from build123d import *

# Parameters (mm, degrees)
SKETCH1_W           = 120
SKETCH1_H           = 48
BOSS_EXTRUDE1_DEPTH = 4
SKETCH2_W           = 14
SKETCH2_H           = 3
BOSS_EXTRUDE2_DEPTH = 5
SKETCH3_R           = 1.7
CUT_EXTRUDE1_DEPTH  = 5
SKETCH4_R           = 3
CUT_EXTRUDE2_DEPTH  = 3


with BuildPart() as part:
    # Sketch1 → Boss-Extrude1 (new body)
    with BuildSketch(Plane(origin=(0, 0, 0), x_dir=(1, 0, 0), z_dir=(0, 1, 0))):
        with Locations((9.738916256, -3.92364532)):
            Rectangle(SKETCH1_W, SKETCH1_H)
    extrude(amount=BOSS_EXTRUDE1_DEPTH)

    # Sketch2 → Boss-Extrude2 (add)
    with BuildSketch(Plane(origin=(0, 4, 0), x_dir=(1, 0, 0), z_dir=(0, 1, 0))):
        Polygon((-50.261083744, 20.07635468), (-17.261083744, 20.07635468), (-17.261083744, 17.07635468), (-47.261083744, 17.07635468), (-47.261083744, -24.92364532), (-17.261083744, -24.92364532), (-17.261083744, -27.92364532), (-50.261083744, -27.92364532), align=None)
        Polygon((69.738916256, 20.07635468), (69.738916256, -27.92364532), (36.738916256, -27.92364532), (36.738916256, -24.92364532), (66.738916256, -24.92364532), (66.738916256, 17.07635468), (36.738916256, 17.07635468), (36.738916256, 20.07635468), align=None)
        with Locations((9.738916256, 18.57635468)):
            Rectangle(SKETCH2_W, SKETCH2_H)
        with Locations((9.738916256, -26.42364532)):
            Rectangle(SKETCH2_W, SKETCH2_H)
    extrude(amount=BOSS_EXTRUDE2_DEPTH)

    # Sketch3 → Cut-Extrude1 (cut)
    with BuildSketch(Plane(origin=(0, 4, 0), x_dir=(1, 0, 0), z_dir=(0, 1, 0))):
        with Locations(Location((4.738916256, -7.848492391, 0), (0, 0, 270))):
            Circle(SKETCH3_R)
        with Locations(Location((-5.261083744, -7.848492391, 0), (0, 0, 270))):
            Circle(SKETCH3_R)
        with Locations(Location((-15.261083744, -7.848492391, 0), (0, 0, 270))):
            Circle(SKETCH3_R)
        with Locations(Location((34.738916256, -7.848492391, 0), (0, 0, 90))):
            Circle(SKETCH3_R)
        with Locations(Location((24.738916256, -7.848492391, 0), (0, 0, 90))):
            Circle(SKETCH3_R)
        with Locations(Location((14.738916256, -7.848492391, 0), (0, 0, 90))):
            Circle(SKETCH3_R)
    extrude(amount=-CUT_EXTRUDE1_DEPTH, mode=Mode.SUBTRACT)

    # Sketch4 → Cut-Extrude2 (cut)
    with BuildSketch(Plane(origin=(0, 4, 0), x_dir=(1, 0, 0), z_dir=(0, 1, 0))):
        with Locations(Location((-15.261083744, -7.848492391, 0), (0, 0, 270))):
            Circle(SKETCH4_R)
        with Locations(Location((-5.261083744, -7.848492391, 0), (0, 0, 270))):
            Circle(SKETCH4_R)
        with Locations(Location((4.738916256, -7.848492391, 0), (0, 0, 270))):
            Circle(SKETCH4_R)
        with Locations(Location((14.738916256, -7.848492391, 0), (0, 0, 270))):
            Circle(SKETCH4_R)
        with Locations(Location((24.738916256, -7.848492391, 0), (0, 0, 270))):
            Circle(SKETCH4_R)
        with Locations(Location((34.738916256, -7.848492391, 0), (0, 0, 270))):
            Circle(SKETCH4_R)
    extrude(amount=-CUT_EXTRUDE2_DEPTH, mode=Mode.SUBTRACT)


solid = part.part
Design review of the part built by this model. Coordinates are the model's own, in mm. A direction names the side the tool comes from. Give positions to 0.01 mm unless a question says otherwise; leave off trailing zeros. Order: outer loops, then holes, each group sorted by start corner. A loop starts at its lowest first (then second) coordinate and runs counter-clockwise, first axis right, second up. Notation, with made-up numbers: (-37, 12) - (-19, 12) arc R7 cw to (-19, 16) - close; hole circle Ø5 at (-39, -1). An arc over 180 degrees is marked (long way). Write item = value, one per line. Start each with the question number.
Q1. To check wall thickness, follow L1, parallel to X at y = 8.75, z = 26; L2, parallel to X at y = 8.25, z = -1.5; L3, parallel to Z at x = 55, y = 4.5. State the ranges of each line that lie inside material, in increasing order. Write a range as from..to.
Q2. We need section A-A on y = 5.5. State the section outline as (x, z) points.
Q3. We need section C-C on x = 60. State the section outline as (y, z) points.
Q4. Tool access review of faces 1 (the face through (16.739, 6, -19)), 2 (the face through (-32, 6, 24.924)), 3 (the face through (-5.91, 0.51, 9.42)): name each direction out of +Z, -Z, +X, -X, +Y, -Y from which nothing blocks a thin tool from reaching the whole face with its end or side.
Q5. Clearance check with flat-ended pins moving along their axes: pin 1 Ø2 at (x, z) = (22.5, 22) entering from +Y; pin 2 Ø5.5 at (x, z) = (4.74, 7.85) entering from +Y. State where each tip first meets the part, or that it passes through.
Q6. We need section B-B on z = 23. State the section outline as (x, y) points, plus the area to 3 significant figures.
Q7. Mouldability with a two-part tool opening along Z and no side actions: class faces 4 (the face through (-7, 1, 9)), 5 (the face through (9, 4, -20.076)), 6 (the face through (-17.261, 6, 26)) as released by +Z, released by -Z, zero draft, split by the parting line, or undercut.
Working result:
q1.L1 = -50.26..-17.26, 2.74..16.74, 36.74..69.74
q1.L2 = -50.26..-47.26, 66.74..69.74
q1.L3 = -20.08..-17.08, 24.92..27.92
q2.outline = (-50.26, -20.08) - (-17.26, -20.08) - (-17.26, -17.08) - (-47.26, -17.08) - (-47.26, 24.92) - (-17.26, 24.92) - (-17.26, 27.92) - (-50.26, 27.92) - close; (2.74, -20.08) - (16.74, -20.08) - (16.74, -17.08) - (2.74, -17.08) - close; (2.74, 24.92) - (16.74, 24.92) - (16.74, 27.92) - (2.74, 27.92) - close; (36.74, -20.08) - (69.74, -20.08) - (69.74, 27.92) - (36.74, 27.92) - (36.74, 24.92) - (66.74, 24.92) - (66.74, -17.08) - (36.74, -17.08) - close
q3.outline = (0, -20.08) - (9, -20.08) - (9, -17.08) - (4, -17.08) - (4, 24.92) - (9, 24.92) - (9, 27.92) - (0, 27.92) - close
q4.face_1 = +Z, -Z, +Y
q4.face_2 = +Y
q4.face_3 = +Y, -Y
q5.pin_1 = 4
q5.pin_2 = 1
q6.outline = (-50.26, 0) - (69.74, 0) - (69.74, 9) - (66.74, 9) - (66.74, 4) - (-47.26, 4) - (-47.26, 9) - (-50.26, 9) - close
q6.area = 510 mm²
q7.face_4 = undercut
q7.face_5 = released by -Z
q7.face_6 = zero draft
